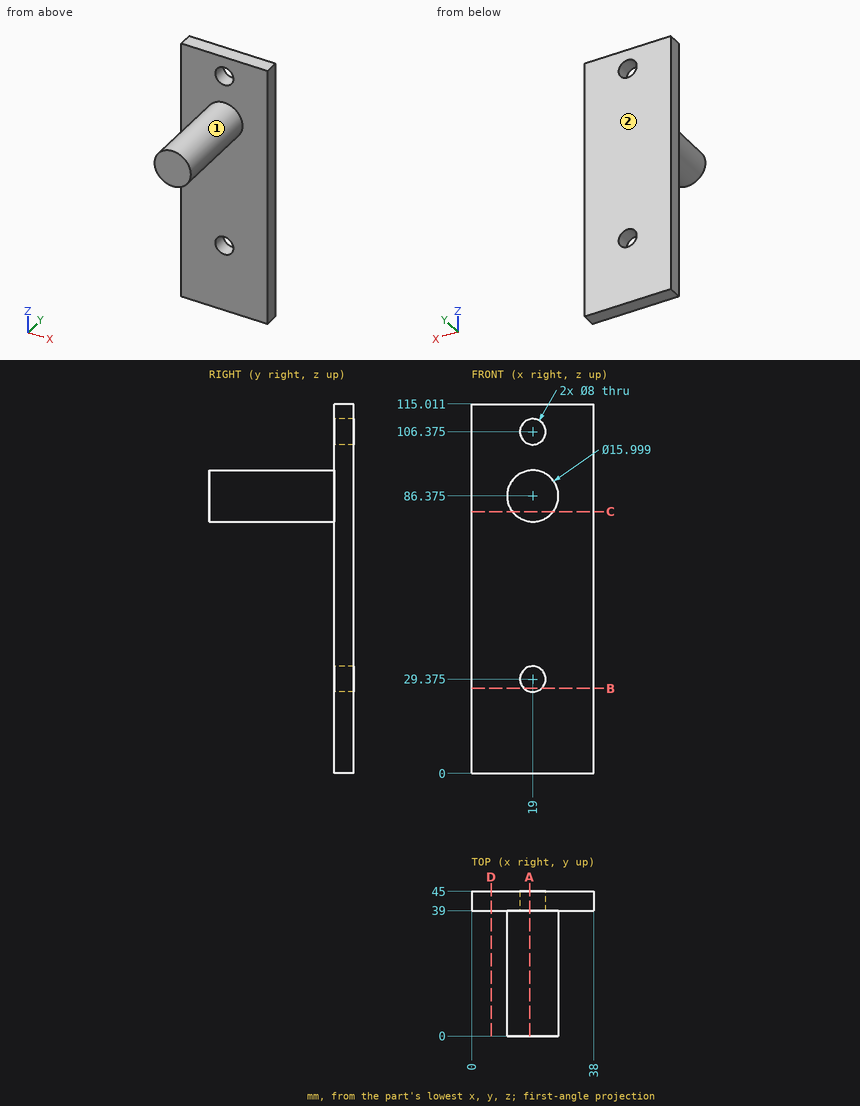
Geometry check sheet. Reference: drawing and pictorial views, mm from the part's lowest x, y, z. A direction names the side the tool comes from. Coordinates: 2 decimals unless noted, no trailing zeros. Order: outer loops, then holes, each group sorted by start corner. A loop starts at its lowest first (then second) coordinate and runs counter-clockwise, first axis right, second up. Notation, with made-up numbers: (48.25, -12) -> (59.25, -12) arc R12 cw to (59.25, 0) -> close; hole circle Ø8 at (71.5, -25). An arc over 180 degrees is marked (long way). Use CSV: the item, a comma, the result in double quotes. Start each with the question number.
Q1. Thickness scan on line 1 along Y through (x, z) = (35.5, 17.5); line 2 along Z through (x, y) = (23.5, 20.5); line 3 along Z through (x, y) = (12.5, 34.5) (1 decimal). Record the ranges inside material, lowest first.
Q2. Section check B-B, the plane z = 26.5. Record the cut outline in (x, y), and give its area (3 significant figures).
Q3. Tool access check on the marked faces 1 and 2. Record the directions out of +Z, -Z, +X, -X, +Y, -Y that give a thin tool (end or side, any length) a straight path to the whole face; none if there is none.
Q4. Depth check by flat-ended pin: P1, Ø10, axis at y = 20, z = 98, coming from the +X side (1 decimal); P2, Ø6, axis at x = 13.5, y = 6.5, coming from the +Z side; P3, Ø8, axis at x = 15, y = 22.5, coming from the -Z side (1 decimal). Enter the tip coordinate at first touch or a pass-through.
Q5. Section check C-C, the plane z = 81.5. Record the cut outline in (x, y).
Q6. Section check A-A, the plane x = 18. Record the cut outline in (y, z).
Q7. Section check D-D, the plane x = 6. Record the cut outline in (y, z).
Returned:
1,line 1,"y = 39 to 45"
1,line 2,"z = 79.76 to 92.99"
1,line 3,"z = 81.7 to 91"
2,outline,"(0, 39) -> (16.22, 39) -> (16.22, 45) -> (0, 45) -> close; (21.78, 39) -> (38, 39) -> (38, 45) -> (21.78, 45) -> close"
2,area,"195 mm^2"
3,face 1,"-Y"
3,face 2,"+Z, -Z, +X, -X, +Y"
4,P1,"stops at x = 23.5"
4,P2,"stops at z = 93.97"
4,P3,"stops at z = 78.4"
5,outline,"(0, 39) -> (12.66, 39) -> (12.66, 0) -> (25.34, 0) -> (25.34, 39) -> (38, 39) -> (38, 45) -> (0, 45) -> close"
6,outline,"(0, 78.44) -> (39, 78.44) -> (39, 33.25) -> (45, 33.25) -> (45, 102.5) -> (39, 102.5) -> (39, 94.31) -> (0, 94.31) -> close; (39, 0) -> (45, 0) -> (45, 25.5) -> (39, 25.5) -> close; (39, 110.25) -> (45, 110.25) -> (45, 115.01) -> (39, 115.01) -> close"
7,outline,"(39, 0) -> (45, 0) -> (45, 115.01) -> (39, 115.01) -> close"
